from build123d import *

# Parameters (mm, degrees)
SALIENTE_EXTRUIR1_DEPTH = 2.5
CROQUIS4_W              = 50
CROQUIS4_H              = 2.5
SALIENTE_EXTRUIR2_DEPTH = 50
REDONDEO2_R             = 3
CROQUIS6_W              = 2.5
CROQUIS6_H              = 42
SALIENTE_EXTRUIR3_DEPTH = 25
REDONDEO3_R             = 2
CORTAR_EXTRUIR1_DEPTH   = 25
CORTAR_EXTRUIR2_START   = -25
CORTAR_EXTRUIR2_DEPTH   = 25
CROQUIS11_W             = 10
CROQUIS11_H             = 22
CORTAR_EXTRUIR3_DEPTH   = 25
CROQUIS12_R             = 2
CORTAR_EXTRUIR4_DEPTH   = 25
CORTAR_EXTRUIR5_START   = -25
CROQUIS13_R             = 2
CORTAR_EXTRUIR5_DEPTH   = 25
CROQUIS14_R             = 2
SALIENTE_EXTRUIR4_DEPTH = 10
CROQUIS15_W             = 7
CROQUIS15_H             = 10
SALIENTE_EXTRUIR5_DEPTH = 40
CROQUIS17_R             = 2
CORTAR_EXTRUIR6_DEPTH   = 50
CROQUIS18_R             = 2
CORTAR_EXTRUIR7_DEPTH   = 50


with BuildPart() as part:
    # Croquis1 → Saliente-Extruir1 (new body)
    with BuildSketch(Plane.XY):
        with BuildLine():
            Line((17, -42.5), (-17, -42.5))
            ThreePointArc((-17, -42.5), (-22.656854249, -40.156854249), (-25, -34.5))
            Line((-25, -34.5), (-25, 42.5))
            Line((-25, 42.5), (25, 42.5))
            Line((25, 42.5), (25, -34.5))
            ThreePointArc((25, -34.5), (22.656854249, -40.156854249), (17, -42.5))
        make_face()
        with BuildLine():
            Line((8, 12.5), (-8, 12.5))
            ThreePointArc((-8, 12.5), (-9.414213562, 13.085786438), (-10, 14.5))
            Line((-10, 14.5), (-10, 30.5))
            ThreePointArc((-10, 30.5), (-9.414213562, 31.914213562), (-8, 32.5))
            Line((-8, 32.5), (8, 32.5))
            ThreePointArc((8, 32.5), (9.414213562, 31.914213562), (10, 30.5))
            Line((10, 30.5), (10, 14.5))
            ThreePointArc((10, 14.5), (9.414213562, 13.085786438), (8, 12.5))
        make_face(mode=Mode.SUBTRACT)
    extrude(amount=SALIENTE_EXTRUIR1_DEPTH)

    # Croquis4 → Saliente-Extruir2 (add)
    with BuildSketch(Plane(origin=(0, 0, 0), x_dir=(-1, 0, 0), z_dir=(0, 0, -1))):
        with Locations((0, 41.25)):
            Rectangle(CROQUIS4_W, CROQUIS4_H)
    extrude(amount=SALIENTE_EXTRUIR2_DEPTH)

    # Redondeo2
    redondeo2_edges = [part.edges().sort_by_distance(p)[0] for p in [
        (0, 42.5, 2.5),
    ]]
    fillet(redondeo2_edges, radius=REDONDEO2_R)

    # Croquis6 → Saliente-Extruir3 (add)
    with BuildSketch(Plane.XZ.offset(-40)):
        with Locations((-23.75, -26)):
            Rectangle(CROQUIS6_W, CROQUIS6_H)
        with Locations((23.75, -26)):
            Rectangle(CROQUIS6_W, CROQUIS6_H)
    extrude(amount=SALIENTE_EXTRUIR3_DEPTH)

    # Redondeo3
    redondeo3_edges = [part.edges().sort_by_distance(p)[0] for p in [
        (0, -42.5, 2.5),
        (22.656854249, -40.156854249, 2.5),
        (25, 2.5, 2.5),
        (-25, 2.5, 2.5),
        (-25, 42.5, -25.25),
        (-25, 41.621320344, 1.621320344),
        (25, 42.5, -25.25),
        (25, 41.621320344, 1.621320344),
        (-22.656854249, -40.156854249, 2.5),
    ]]
    fillet(redondeo3_edges, radius=REDONDEO3_R)

    # Croquis7 → Cortar-Extruir1 (cut)
    with BuildSketch(Plane(origin=(25, 0, 0), x_dir=(0, 0, -1), z_dir=(1, 0, 0))):
        Polygon((39, 15), (47, 25), (47, 15), align=None)
        with BuildLine():
            Line((5, 18), (5, 15))
            Line((5, 15), (8, 15))
            ThreePointArc((8, 15), (5.878679656, 15.878679656), (5, 18))
        make_face()
    extrude(amount=-CORTAR_EXTRUIR1_DEPTH, mode=Mode.SUBTRACT)

    # Croquis8 → Cortar-Extruir2 (cut)
    with BuildSketch(Plane.ZY.offset(25).offset(CORTAR_EXTRUIR2_START)):
        Polygon((-39, 15), (-47, 15), (-47, 25), align=None)
        with BuildLine():
            Line((-5, 18), (-5, 15))
            Line((-5, 15), (-8, 15))
            ThreePointArc((-8, 15), (-5.878679656, 15.878679656), (-5, 18))
        make_face()
    extrude(amount=CORTAR_EXTRUIR2_DEPTH, mode=Mode.SUBTRACT)

    # Croquis11 → Cortar-Extruir3 (cut)
    with BuildSketch(Plane.XZ.offset(-40)):
        with Locations((0, -25)):
            Rectangle(CROQUIS11_W, CROQUIS11_H)
    extrude(amount=-CORTAR_EXTRUIR3_DEPTH, mode=Mode.SUBTRACT)

    # Croquis12 → Cortar-Extruir4 (cut)
    with BuildSketch(Plane.ZY.offset(25)):
        with Locations(Location((-25.25, 33, 0), (0, 0, 270))):
            Circle(CROQUIS12_R)
    extrude(amount=-CORTAR_EXTRUIR4_DEPTH, mode=Mode.SUBTRACT)

    # Croquis13 → Cortar-Extruir5 (cut)
    with BuildSketch(Plane(origin=(25, 0, 0), x_dir=(0, 0, -1), z_dir=(1, 0, 0)).offset(CORTAR_EXTRUIR5_START)):
        with Locations(Location((25.25, 33, 0), (0, 0, 270))):
            Circle(CROQUIS13_R)
    extrude(amount=CORTAR_EXTRUIR5_DEPTH, mode=Mode.SUBTRACT)

    # Croquis14 → Saliente-Extruir4 (add)
    with BuildSketch(Plane(origin=(0, 42.5, 0), x_dir=(1, 0, 0), z_dir=(0, 1, 0))):
        with Locations(Location((-10, 25, 0), (0, 0, 90))):
            Circle(CROQUIS14_R)
        with Locations(Location((10, 25, 0), (0, 0, 90))):
            Circle(CROQUIS14_R)
    extrude(amount=SALIENTE_EXTRUIR4_DEPTH)

    # Croquis15 → Saliente-Extruir5 (add)
    with BuildSketch(Plane(origin=(0, 0, 0), x_dir=(-1, 0, 0), z_dir=(0, 0, -1))):
        with Locations((-7, -19.5)):
            Rectangle(CROQUIS15_W, CROQUIS15_H)
        with Locations((7, -19.5)):
            Rectangle(CROQUIS15_W, CROQUIS15_H)
    extrude(amount=SALIENTE_EXTRUIR5_DEPTH)

    # Croquis17 → Cortar-Extruir6 (cut)
    with BuildSketch(Plane(origin=(0, -14.5, 0), x_dir=(1, 0, 0), z_dir=(0, 1, 0))):
        with Locations(Location((-7, 35, 0), (0, 0, 270))):
            Circle(CROQUIS17_R)
    extrude(amount=-CORTAR_EXTRUIR6_DEPTH, mode=Mode.SUBTRACT)

    # Croquis18 → Cortar-Extruir7 (cut)
    with BuildSketch(Plane(origin=(0, -14.5, 0), x_dir=(1, 0, 0), z_dir=(0, 1, 0))):
        with Locations(Location((7, 35, 0), (0, 0, 270))):
            Circle(CROQUIS18_R)
    extrude(amount=-CORTAR_EXTRUIR7_DEPTH, mode=Mode.SUBTRACT)


solid = part.part
Input: part model. Units: mm. Frame: model coordinates. A direction names the side the tool comes from. Coordinates: 2 decimals unless noted, no trailing zeros. Loops run counter-clockwise (first coordinate to the right, second up) from the corner with the lowest first, then second, coordinate; pieces in that order, holes last. Notation, with made-up numbers: (22, 41.5) -> (66, 41.5) arc R9 cw to (66, 47.5) -> close; hole circle Ø11 at (39.25, 85.5). An arc over 180 degrees is marked (long way). Write each question's results on one line, items separated by ' | '. Start each with the question number.
Q1. Pin query (flat end, axial travel): pin 1 (7.5 mm diameter, centred on x = -5.5, z = -21.5, fed in from -Y); pin 2 (12 mm diameter, centred on x = -12.5, y = 5, fed in from -Z); pin 3 (3 mm diameter, centred on x = 23, z = -29.5, fed in from -Y). Return the tip coordinate at first contact, or that it passes through.
Q2. Pull-direction query (Z, two-part tool) for faces 1 (the flat face through (0, 0, 2.5)), 2 (the cylindrical face through (8.648, 47.43, -23.526)), 3 (the flat face through (7, -14.5, -20)), 4 (the flat face through (-5, 41, -25)); classes: released by +Z, released by -Z, zero draft, split by the parting line, or undercut.
Q3. Reachability of faces 5 (the flat face through (7, -24.5, -20)), 6 (the flat face through (-7, -14.5, -20)), 7 (the cylindrical face through (-9.4, 13.07, 1.23)) from +Z, -Z, +X, -X, +Y, -Y: full face, straight path, thin tool, end or side. Return the list, or none.
Q4. Section A-A, the plane z = -3. Return the cut outline in (x, y).
Q5. Section B-B, the plane x = 7. Return the cut outline in (y, z).
Q6. Section D-D, the plane y = 13.5. Return the cut outline in (x, z), plus the area to 3 significant figures.
Q7. Ray query, line 1 (Z direction, x = 23, y = 33); line 2 (Y direction, x = 10, z = -14.5); line 3 (X direction, y = 26, z = -6.5). Return the intervals inside material, ascending. Write a range as from..to.
Q8. Section C-C, the plane y = -21. Return the cut outline in (x, z).
Found:
1) pin 1: y = -24.5 | pin 2: z = 0 | pin 3: y = 15
2) face 1: released by +Z | face 2: split by the parting line | face 3: zero draft | face 4: undercut
3) face 5: -Z, +X, -X, -Y | face 6: -Z, +X, -X | face 7: +Z, -Z
4) outline: (-25, 40) -> (25, 40) -> (25, 40.5) arc R2 ccw to (23, 42.5) -> (-23, 42.5) arc R2 ccw to (-25, 40.5) -> close; (-10.5, -24.5) -> (-3.5, -24.5) -> (-3.5, -14.5) -> (-10.5, -14.5) -> close; (3.5, -24.5) -> (10.5, -24.5) -> (10.5, -14.5) -> (3.5, -14.5) -> close
5) outline: (-42.5, 0) -> (-24.5, 0) -> (-24.5, -33) -> (-14.5, -33) -> (-14.5, 0) -> (12.5, 0) -> (12.5, 2.5) -> (-40.5, 2.5) arc R2 ccw to (-42.5, 0.5) -> close; (-24.5, -40) -> (-14.5, -40) -> (-14.5, -37) -> (-24.5, -37) -> close; (32.5, 0) -> (40, 0) -> (40, -50) -> (42.5, -50) -> (42.5, -0.5) arc R3 ccw to (39.5, 2.5) -> (32.5, 2.5) -> close
6) outline: (-25, 0) -> (-9.73, 0) -> (-9.73, 2.5) -> (-23, 2.5) arc R2 ccw to (-25, 0.5) -> close; (9.73, 0) -> (25, 0) -> (25, 0.5) arc R2 ccw to (23, 2.5) -> (9.73, 2.5) -> close | area: 74.6 mm2
7) line 1: -47..-27.25, -23.25..-5, 0..2.5 | line 2: -24.5..-14.5, 40..42.5 | line 3: -25..-22.5, 22.5..25
8) outline: (-25, 0) -> (-10.5, 0) -> (-10.5, -40) -> (-3.5, -40) -> (-3.5, 0) -> (3.5, 0) -> (3.5, -40) -> (10.5, -40) -> (10.5, 0) -> (25, 0) -> (25, 0.5) arc R2 ccw to (23, 2.5) -> (-23, 2.5) arc R2 ccw to (-25, 0.5) -> close; hole circle Ø4 at (-7, -35); hole circle Ø4 at (7, -35)
